```python
from build123d import *

# Parameters (mm, degrees)
BOSS_EXTRUDE1_DEPTH = 355.6
SKETCH8_W           = 736.392149349
SKETCH8_H           = 355.6
CUT_EXTRUDE2_DEPTH  = 5.08
CUT_EXTRUDE4_REACH  = 892.111
SKETCH12_R          = 3.9624


with BuildPart() as part:
    # Sketch2 → Boss-Extrude1 (new body)
    with BuildSketch(Plane(origin=(0, 0, 0), x_dir=(1, 0, 0), z_dir=(0, 1, 0))):
        Polygon((-328.93, -373.38), (328.93, -373.38), (328.93, 373.38), (0, 297.18), (-328.93, 373.38), align=None)
        Polygon((-323.85, -368.3), (323.85, -368.3), (323.85, 368.159900717), (0, 293.136734694), (-323.85, 368.159900717), align=None, mode=Mode.SUBTRACT)
    extrude(amount=BOSS_EXTRUDE1_DEPTH)

    # Sketch8 → Cut-Extrude2 (cut)
    with BuildSketch(Plane(origin=(328.93, 0, 0), x_dir=(0, 0, -1), z_dir=(1, 0, 0))):
        with Locations((0.86314386, 177.8)):
            Rectangle(SKETCH8_W, SKETCH8_H)
    extrude(amount=-CUT_EXTRUDE2_DEPTH, mode=Mode.SUBTRACT)

    # Cut-Extrude4: up to this plane
    cut_extrude4_end = Plane(origin=(328.93, 355.6, -373.38), z_dir=(0.22568355160076956, 0, 0.9742006644099884))
    # Sketch12 → Cut-Extrude4 (cut, up to the surface)
    with BuildSketch(Plane.XY.offset(373.38), mode=Mode.PRIVATE) as cut_extrude4_sk1:
        with Locations(Location((315.000794765, 6.297541098, 0), (0, 0, 180))):
            Circle(SKETCH12_R)
    cut_extrude4_tool1 = split(extrude(cut_extrude4_sk1.sketch, amount=-CUT_EXTRUDE4_REACH, mode=Mode.PRIVATE), bisect_by=cut_extrude4_end, keep=Keep.BOTH, mode=Mode.PRIVATE)
    add(cut_extrude4_tool1.solids().sort_by_distance((315.000795, 6.297541, 373.38))[0], mode=Mode.SUBTRACT)


solid = part.part
```
Can you work these out from the model? Positions are in its coordinate system, mm. A direction names the side the tool comes from. Give positions to 0.01 mm unless a question says otherwise; leave off trailing zeros. Loops run counter-clockwise (first coordinate to the right, second up) from the corner with the lowest first, then second, coordinate; pieces in that order, holes last. Notation, with made-up numbers: M 81,-18 L 134,-18 A22 ccw 134,-7 Z; hole C 31.5,-36 d6. An arc over 180 degrees is marked long. One line per question, with ' | ' between items. Start each with the question number.
Q1. If we mould it in two halves opening along X, with no side actions, what happens to faces 1 (the flat face through (-162.162, 175.311, -334.747)), 2 (the flat face through (164.192, 175.311, -331.173)), 3 (the flat face through (-328.93, 175, -5)), 4 (the flat face through (166.768, 175.311, -335.813))? For each: +X half, -X half, draft (parallel to the pull), parting line (faces both ways), or undercut.
Q2. For pin 1 Ø4 at (x, y) = (92.5, 241) entering from -Z; pin 2 Ø3 at (y, z) = (199.5, -286) entering from +X; pin 3 Ø12 at (x, y) = (241, 107.5) entering from -Z, each with a flat end and sliding along its axis, tell me the tip position at first contact or that it passes through.
Q3. For faces 5 (the flat face through (-5, 175, 368.3)), 6 (the flat face through (-5, 175, 373.38)), which set-ups out of +Z, -Z, +X, -X, +Y, -Y let a thin tool reach every point of the face, with its end or its side?
Q4. If I drill on line 1 (X direction, y = 199.5, z = 21.5); line 2 (Z direction, x = -19, y = 176); line 3 (Z direction, x = -195, y = 240), over which ranges is the centre line in solid material (lowest first)? Write a range as from..to.
Q5. If we section it at B-B (x = -11.5): Please give me the cut outline in (y, z), plus the area to 3 significant figures.
Q6. If we section it at C-C (z = 93.5): Please give me the cut outline in (x, y), plus the area to 3 significant figures.
Q7. If we section it at A-A (y = 282): Please give me the cut outline in (x, z).
Computed:
1) face 1: undercut | face 2: +X half | face 3: -X half | face 4: undercut
2) pin 1: stops at z = -319.07 | pin 2: stops at x = -323.85 | pin 3: stops at z = -354.4
3) face 5: +Y, -Y | face 6: +Z, +X, -X, +Y, -Y
4) line 1: x = -328.93..-323.85 | line 2: z = -301.58..-297.54, 368.3..373.38 | line 3: z = -342.35..-338.31, 368.3..373.38
5) outline: M 0,-299.84 L 355.6,-299.84 L 355.6,-295.8 L 0,-295.8 Z; M 0,368.3 L 355.6,368.3 L 355.6,373.38 L 0,373.38 Z | area: 3,240 mm²
6) outline: M -328.93,0 L -323.85,0 L -323.85,355.6 L -328.93,355.6 Z | area: 1,810 mm²
7) outline: M -328.93,-373.38 L 0,-297.18 L 328.93,-373.38 L 328.93,-369.06 L 323.85,-369.06 L 323.85,-368.16 L 0,-293.14 L -323.85,-368.16 L -323.85,368.3 L 323.85,368.3 L 323.85,367.33 L 328.93,367.33 L 328.93,373.38 L -328.93,373.38 Z
